Could you check a few things on this model? Use its own coordinates, in mm. A direction names the side the tool comes from. Coordinates: 2 decimals unless noted, no trailing zeros. Order: outer loops, then holes, each group sorted by start corner. A loop starts at its lowest first (then second) coordinate and runs counter-clockwise, first axis right, second up.
```python
from build123d import *

# Parameters (mm, degrees)
CUT_EXTRUDE1_START = 15.8749999
CUT_EXTRUDE1_DEPTH = 2.0828001


with BuildPart() as part:
    # Sketch2 → Revolve1 (revolve)
    with BuildSketch(Plane(origin=(0, 0, 0), x_dir=(0, 0, -1), z_dir=(1, 0, 0)), mode=Mode.PRIVATE) as revolve1_sk:
        with BuildLine():
            Line((17.9578, 0), (17.9578, 1.4874875))
            Line((17.9578, 1.4874875), (17.3624875, 2.0828))
            Line((17.3624875, 2.0828), (-13.7922, 2.0828))
            Line((-13.7922, 2.0828), (-13.7922, 3.22072))
            ThreePointArc((-13.7922, 3.22072), (-13.8532038, 3.3679962), (-14.00048, 3.429))
            Line((-14.00048, 3.429), (-17.74952, 3.429))
            ThreePointArc((-17.74952, 3.429), (-17.8967962, 3.3679962), (-17.9578, 3.22072))
            Line((-17.9578, 3.22072), (-17.9578, 1.7859375))
            Line((-17.9578, 1.7859375), (-15.875, 1.7859375))
            Line((-15.875, 1.7859375), (-14.843888504, 0))
            Line((-14.843888504, 0), (17.9578, 0))
        make_face()
    revolve(revolve1_sk.sketch.rotate(Axis((0, 0, -17.9578), (0, 0, 1)), 90), axis=Axis((0, 0, -17.9578), (0, 0, 1)))

    # Cut-Extrude1: read off the stored shape, not the designer's step
    # Cut-Extrude1 outline → Cut-Extrude1 (cut)
    with BuildSketch(Plane.XY.offset(CUT_EXTRUDE1_START)):
        with BuildLine():
            Line((0.892981609, 1.54665982), (0, 2.062222993))
            Line((0, 2.062222993), (-0.892981609, 1.54665982))
            ThreePointArc((-0.892981609, 1.54665982), (0, 1.7859375), (0.892981609, 1.54665982))
        make_face()
        with BuildLine():
            ThreePointArc((-1.7859375, 0), (-1.546670957, 0.89296232), (-0.892981609, 1.54665982))
            Line((-0.892981609, 1.54665982), (-1.7859375, 1.031111496))
            Line((-1.7859375, 1.031111496), (-1.7859375, 0))
        make_face()
        with BuildLine():
            Line((1.7859375, 1.031111496), (0.892981609, 1.54665982))
            ThreePointArc((0.892981609, 1.54665982), (1.546670957, 0.89296232), (1.7859375, 0))
            Line((1.7859375, 0), (1.7859375, 1.031111496))
        make_face()
        with BuildLine():
            ThreePointArc((-0.892981609, -1.54665982), (-1.546670957, -0.89296232), (-1.7859375, 0))
            Line((-1.7859375, 0), (-1.7859375, -1.031111496))
            Line((-1.7859375, -1.031111496), (-0.892981609, -1.54665982))
        make_face()
        with BuildLine():
            Line((1.7859375, -1.031111496), (1.7859375, 0))
            ThreePointArc((1.7859375, 0), (1.546670957, -0.89296232), (0.892981609, -1.54665982))
            Line((0.892981609, -1.54665982), (1.7859375, -1.031111496))
        make_face()
        with BuildLine():
            ThreePointArc((0.892981609, -1.54665982), (0, -1.7859375), (-0.892981609, -1.54665982))
            Line((-0.892981609, -1.54665982), (0, -2.062222993))
            Line((0, -2.062222993), (0.892981609, -1.54665982))
        make_face()
    extrude(amount=CUT_EXTRUDE1_DEPTH, mode=Mode.SUBTRACT)

    # Cut-Extrude1 2 outline → Cut-Extrude1 2 (revolve)
    with BuildSketch(Plane.XZ):
        Polygon((2.062223129, 16.034513582), (1.785937457, 15.874999975), (2.062222993, 15.8749999), align=None)
    revolve(axis=Axis((0, 0, 0), (0, 0, 1)))

    # Cut-Extrude2 cone 1 section (on through the dimple's axis) → Cut-Extrude2 (revolve, cut)
    with BuildSketch(Plane(origin=(0, 0, 17.9578), x_dir=(0, -1, 0), z_dir=(1, 0, 0))):
        Polygon((0, 0), (2.255305827, 0), (0, 1.302101426), align=None)
    revolve(axis=Axis((0, 0, 17.9578), (0, 0, -1)), mode=Mode.SUBTRACT)


solid = part.part
```
Item 1: For pin 1 Ø0.6 at (y, z) = (-0.5, 17) entering from -X; pin 2 Ø1 at (y, z) = (1, -12.5) entering from -X; pin 3 Ø4 at (y, z) = (-1, 3.5) entering from +X, each with a flat end and sliding along its axis, tell me the tip position at first contact or that it passes through.
Item 2: I need wall thicknesses on line 1 (Z direction, x = 2.75, y = -1); line 2 (Y direction, x = 0, z = -3); line 3 (Z direction, x = -1, y = -1). Which ranges of each line are inside material? Lowest first, please.
Item 3: Which directions (+Z, -Z, +X, -X, +Y, -Y) give clear straight access to the entire face, cutting with the end or side of a thin tool? Please do faces 4 (the face through (-1.987, -0.626, -1.567)), 5 (the face through (-1.4, 2.1, 17.958)), 6 (the face through (1.786, 0, 17)).
Item 4: Thinking about a two-plate mould opening in Y: for faces 1 (the face through (0, 0, -17.958)), 2 (the face through (0.74, 3.35, 15.9)), 3 (the face through (-1.786, 0, 17)), which applies, +Y half, -Y half, draft (parallel to the pull), parting line (faces both ways), or undercut?
Item 5: Suppose I cut it at A-A (z = -15). List the corners of the cut face in (x, y) for me.
Geometry results:
1. pin 1: stops at x = -3.42
1. pin 2: stops at x = -2.02
1. pin 3: stops at x = 2.08
2. line 1: z = 13.79 to 17.96
2. line 2: y = -2.08 to 2.08
2. line 3: z = -17.96 to 15.66
3. face 4: -Z
3. face 5: +Z, +X, -X, +Y, -Y
3. face 6: +Z
4. face 1: draft
4. face 2: parting line
4. face 3: undercut
5. outline: circle Ø4.17 at (0, 0)
